Work out the finished part from the listing and answer in its coordinate system (mm). Face numbers are marked on the shaded views. A direction names the side the tool comes from. Round coordinates to 2 decimals unless told otherwise and drop trailing zeros. Write each loop counter-clockwise with the first axis right and the second up, starting at its lowest first coordinate (ties: lowest second). Pieces come first, ordered by that corner, then holes. Notation, with made-up numbers: (84.25, -10.75) -> (88.25, -10.75) arc R20 ccw to (88.25, -3.75) -> close; hole circle Ø4 at (23.5, 24). An arc over 180 degrees is marked (long way). One line per item, written item: value.
```python
from build123d import *

# Parameters (mm, degrees)
EXTRUDE_1_DEPTH          = 1
SKETCH_2_R               = 2.5
EXTRUDE_2_DEPTH          = 3
SKETCH_3_R               = 1
CUT_EXTRUDE_1_DEPTH      = 14.280344359
SKETCH_4_R               = 2
CUT_EXTRUDE_2_DEPTH      = 0.5
CUT_EXTRUDE_3_DEPTH      = 14.014128718
CUT_EXTRUDE_3_DEPTH_BACK = 14.014128718
M1_2X0_25_1_D            = 0.95
M1_2X0_25_1_CSINK_D      = 1.25
M1_2X0_25_1_CSINK_ANGLE  = 90


with BuildPart() as part:
    # 草图1 → 凸台-拉伸1 (new body)
    with BuildSketch(Plane.XY):
        with BuildLine():
            ThreePointArc((5.387901985, -3.996312325), (8.863269777, -1.562833599), (6.429791051, 1.912534193))
            Line((6.429791051, 1.912534193), (3, 2.517298894))
            Line((3, 2.517298894), (3, 6))
            ThreePointArc((3, 6), (0, 9), (-3, 6))
            Line((-3, 6), (-3, 0))
            ThreePointArc((-3, 0), (-2.298133329, -1.928362829), (-0.520944533, -2.954423259))
            Line((-0.520944533, -2.954423259), (5.387901985, -3.996312325))
        make_face()
        with BuildLine():
            ThreePointArc((0.520944516, 2.954423262), (0.26146722, 2.988584095), (1e-09, 3))
            Line((0, 3), (0, 3.046279836))
            Line((0, 3.046279836), (0.520944516, 2.954423262))
        make_face(mode=Mode.SUBTRACT)
    extrude(amount=EXTRUDE_1_DEPTH)

    # 草图2 → 凸台-拉伸2 (add)
    with BuildSketch(Plane(origin=(0, 0, 0), x_dir=(-1, 0, 0), z_dir=(0, 0, -1))):
        with Locations(Location((0, 0, 0), (0, 0, 180))):
            Circle(SKETCH_2_R)
    extrude(amount=EXTRUDE_2_DEPTH)

    # 草图3 → 切除-拉伸1 (cut, through all)
    with BuildSketch(Plane(origin=(0, 0, -3), x_dir=(-1, 0, 0), z_dir=(0, 0, -1))):
        Circle(SKETCH_3_R)
    extrude(amount=-CUT_EXTRUDE_1_DEPTH, mode=Mode.SUBTRACT)

    # 草图4 → 切除-拉伸2 (cut)
    with BuildSketch(Plane.XY.offset(1)):
        Circle(SKETCH_4_R)
    extrude(amount=-CUT_EXTRUDE_2_DEPTH, mode=Mode.SUBTRACT)

    # 草图5 → 切除-拉伸3 (cut, two sides: drawn at the far end of the back side and taken through both)
    with BuildSketch(Plane(origin=(0, 0, 0), x_dir=(1, 0, 0), z_dir=(0, 1, 0)).offset(-CUT_EXTRUDE_3_DEPTH_BACK)):
        Polygon((-2.5, 3), (2.5, 0.113248654), (2.5, 3), align=None)
    extrude(amount=CUT_EXTRUDE_3_DEPTH + CUT_EXTRUDE_3_DEPTH_BACK, mode=Mode.SUBTRACT)

    # M1.2x0.25 螺纹孔1 (through all)
    with Locations(Plane.XY.offset(1)):
        with Locations((0, 6), (5.908846518, -1.041889066)):
            CounterSinkHole(M1_2X0_25_1_D / 2, M1_2X0_25_1_CSINK_D / 2, counter_sink_angle=M1_2X0_25_1_CSINK_ANGLE)


solid = part.part
```
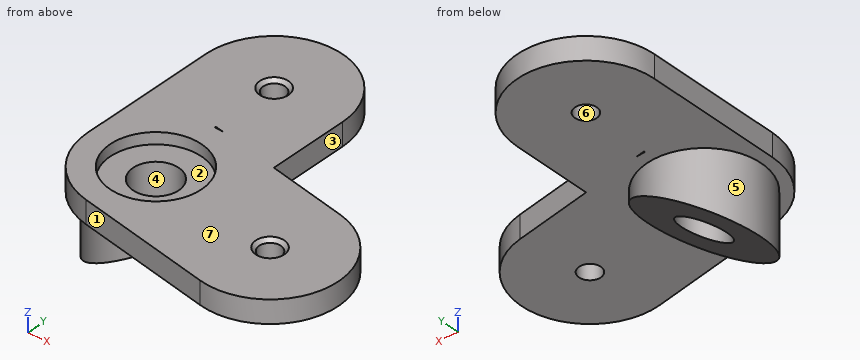
(1) Find section D-D on z = -1.1. Give the vertices of the cut face in (x, y), plus the area to 3 significant figures.
Reported:
outline: (0.79, -2.37) -> (0.79, -0.61) arc R1 cw (long way) to (0.79, 0.61) -> (0.79, 2.37) arc R2.5 ccw (long way) to start
area: 10.7 mm2
(2) Flat-ended cylindrical pins translate along their axes: pin 1 Ø0.8 at (y, z) = (4, 0.5) entering from +X; pin 2 Ø2.5 at (x, y) = (0, 0) entering from +Z; pin 3 Ø1.5 at (x, z) = (0.5, -2.5) entering from -Y; pin 4 Ø3.5 at (x, y) = (1, 1.5) entering from -Z. Find the tip coordinate at first contact, or state that the pin passes through.
Reported:
pin 1: stops at x = 3
pin 2: stops at z = 0.5
pin 3: passes through
pin 4: stops at z = -1.99
(3) For a pull along X with two mould halves and no side action, classify the marked faces 4, 5, 6 and 7 as pulls with the +X half, pulls with the -X half, needs draft (parallel to the pull), parting line crosses it, or undercut.
Reported:
face 4: undercut
face 5: parting line crosses it
face 6: undercut
face 7: needs draft
(4) A tool of negligible diameter and unlimited length cuts with its end or side. For the marked faces 1, 2 and 3, from which of +Z, -Z, +X, -X, +Y, -Y can it reach the whole face along a straight path? Write none if from no direction.
Reported:
face 1: +Z, -Z, -X, -Y
face 2: +Z
face 3: +Z, -Z, +X, +Y
(5) Find section B-B on y = 3.25. Give the vertices of the cut face in (x, z).
Reported:
outline: (-3, 0) -> (3, 0) -> (3, 1) -> (-3, 1) -> close
(6) Consider probe 1 along X at (y, z) = (6, 0.35) (3 decimals); probe 2 along Y at (x, z) = (0, -0.35); probe 3 along Z at (x, y) = (2.25, -2.5). Determine where each line is inside the solid, lowest interval first.
Reported:
probe 1: x = -3 to -0.475, 0.475 to 3
probe 2: y = -2.5 to -1, 1 to 2.5
probe 3: z = 0 to 1
(7) Find section C-C on x = 1.5. Give the vertices of the cut face in (y, z).
Reported:
outline: (-3.31, 0) -> (-2, 0) -> (-2, -0.69) -> (2, -0.69) -> (2, 0) -> (8.6, 0) -> (8.6, 1) -> (1.32, 1) -> (1.32, 0.5) -> (-1.32, 0.5) -> (-1.32, 1) -> (-3.31, 1) -> close
(8) Find section A-A on z = 0.2. Give the vertices of the cut face in (x, y) (3 decimals).
Reported:
outline: (-3, 0) arc R3 ccw to (-0.521, -2.954) -> (5.388, -3.996) arc R3 ccw to (6.43, 1.913) -> (3, 2.517) -> (3, 6) arc R3 ccw to (-3, 6) -> close; hole circle Ø2 at (0, 0); hole circle Ø0.95 at (0, 6); hole (0, 3) arc R3 cw to (0.521, 2.954) -> (0, 3.046) -> close; hole circle Ø0.95 at (5.909, -1.042)
